from build123d import *

# Parameters (mm, degrees)
BOSS_EXTRUDE1_DEPTH = 2.54
SKETCH3_W           = 9.6012
SKETCH3_H           = 10.7188
SKETCH3_W_2         = 10.0076
SKETCH3_H_2         = 14.5034
BOSS_EXTRUDE2_DEPTH = 4.572
SKETCH4_R           = 0.635
CUT_EXTRUDE1_DEPTH  = 3.54
SKETCH5_R           = 0.99949
CUT_EXTRUDE2_DEPTH  = 3.54


with BuildPart() as part:
    # Sketch1 → Boss-Extrude1 (new body)
    with BuildSketch(Plane(origin=(0, 0, 0), x_dir=(1, 0, 0), z_dir=(0, 1, 0))):
        Polygon((-47.9425, 45.085), (-39.6875, 45.085), (-39.6875, 57.785), (39.6875, 57.785), (39.6875, 45.085), (47.9425, 45.085), (47.9425, -45.085), (39.6875, -45.085), (39.6875, -57.785), (-39.6875, -57.785), (-39.6875, -45.085), (-47.9425, -45.085), align=None)
    extrude(amount=BOSS_EXTRUDE1_DEPTH)

    # Sketch3 → Boss-Extrude2 (add)
    with BuildSketch(Plane(origin=(0, 0, 0), x_dir=(1, 0, 0), z_dir=(0, 1, 0))):
        with Locations((-10.1473, -19.177)):
            Rectangle(SKETCH3_W, SKETCH3_H)
        with Locations((-8.7757, 23.368)):
            Rectangle(SKETCH3_W_2, SKETCH3_H_2)
    extrude(amount=BOSS_EXTRUDE2_DEPTH)

    # Sketch4 → Cut-Extrude1 (cut, through all)
    with BuildSketch(Plane(origin=(0, 2.54, 0), x_dir=(1, 0, 0), z_dir=(0, 1, 0))):
        with Locations((4.2545, -34.417)):
            Circle(SKETCH4_R)
        with Locations((-23.6855, -34.417)):
            Circle(SKETCH4_R)
        with Locations((-9.7155, -3.937)):
            Circle(SKETCH4_R)
        with Locations((4.2545, 11.43)):
            Circle(SKETCH4_R)
        with Locations((-23.6855, 11.43)):
            Circle(SKETCH4_R)
        with Locations((-9.7155, 41.91)):
            Circle(SKETCH4_R)
    extrude(amount=-CUT_EXTRUDE1_DEPTH, mode=Mode.SUBTRACT)

    # Sketch5 → Cut-Extrude2 (cut, through all)
    with BuildSketch(Plane(origin=(0, 2.54, 0), x_dir=(1, 0, 0), z_dir=(0, 1, 0))):
        with Locations((42.8625, -40.005)):
            Circle(SKETCH5_R)
        with Locations((42.8625, 40.005)):
            Circle(SKETCH5_R)
        with Locations((-42.8625, -40.005)):
            Circle(SKETCH5_R)
        with Locations((-42.8625, 40.005)):
            Circle(SKETCH5_R)
    extrude(amount=-CUT_EXTRUDE2_DEPTH, mode=Mode.SUBTRACT)


solid = part.part
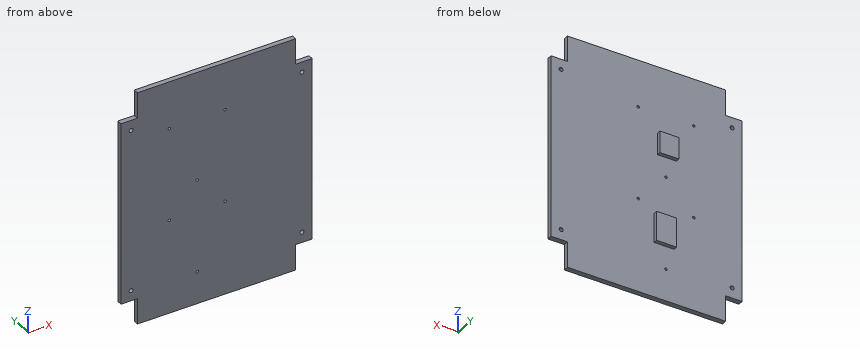
Input: part model. Units: mm. Frame: model coordinates. Give positions to 0.01 mm unless a question says otherwise; leave off trailing zeros. Order: outer loops, then holes, each group sorted by start corner. A loop starts at its lowest first (then second) coordinate and runs counter-clockwise, first axis right, second up.
Q1. Section B-B on x = 17. Output: boundary loops of the cut face in (y, z) (3 decimals), and give its area (3 significant figures).
Checked values:
outline: (0, -57.785) - (2.54, -57.785) - (2.54, 57.785) - (0, 57.785) - close
area: 294 mm2
Q2. Section A-A on y = 3.7. Output: boundary loops of the cut face in (x, z).
Checked values:
outline: (-14.95, 13.82) - (-5.35, 13.82) - (-5.35, 24.54) - (-14.95, 24.54) - close; (-13.78, -30.62) - (-3.77, -30.62) - (-3.77, -16.12) - (-13.78, -16.12) - close
Q3. Section C-C on z = 9. Output: boundary loops of the cut face in (x, y).
Checked values:
outline: (-47.94, 0) - (47.94, 0) - (47.94, 2.54) - (-47.94, 2.54) - close
Q4. Contact query for flat-ended pins moving along their axis: pin 1 Ø3 at (x, z) = (19.5, 0.5) entering from +Y; pin 2 Ø6 at (x, z) = (-16.5, 27.5) entering from -Y; pin 3 Ø1.6 at (x, y) = (-8, 3.5) entering from +Z; pin 4 Ø2 at (x, y) = (-43, 1.5) entering from -Z (3 decimals). Output: stop coordinate, or through.
Checked values:
pin 1: stops at y = 2.54
pin 2: stops at y = 0
pin 3: stops at z = 24.54
pin 4: stops at z = -45.085
Q5. Ray query, probe 1 along X at (y, z) = (1.4, -11.43); probe 2 along Y at (x, z) = (-27.5, 42.5); probe 3 along Z at (x, y) = (-44, 1.6) (3 decimals). Return the intervals inside material, ascending.
Checked values:
probe 1: x = -47.94 to -24.32, -23.05 to 3.62, 4.89 to 47.94
probe 2: y = 0 to 2.54
probe 3: z = -45.085 to 45.085
